Autodesk Inventor part; units mm, degrees
ref_plane "YZ Plane" through (0, 0, 0) normal (1, 0, 0) x (0, 1, 0)
ref_plane "XZ Plane" through (0, 0, 0) normal (0, 1, 0) x (-1, 0, 0)
ref_plane "XY Plane" through (0, 0, 0) normal (0, 0, 1) x (1, 0, 0)
sketch "Sketch4" plane through (0, 0, 0) normal (0, 0, 1) x (1, 0, 0)
  arc A0 (0.0635, 6.3497) -> (6.3497, 0.0635) centre (0, 0) ccw
  arc A1 (-1.1235, 7.5367) -> (7.5367, -1.1235) centre (0, 0) ccw
  line L0 (0, 0) -> (0, 7.9375) construction
  line L1 (0.0635, 6.3497) -> (6.3497, 0.0635) construction
  line L2 (0.0635, 6.3497) -> (-1.1235, 7.5367)
  line L3 (6.3497, 0.0635) -> (7.5367, -1.1235)
  circle A2 centre (0, 0) radius 6.35
  dimension "d10" = 12.7
  dimension "d11" = 1.27
  dimension "d12" = 45
  dimension "d13" = 8.89
extrude "Extrusion3" add sketch "Sketch4" along normal mid plane 35.56 contours A0 L3 A1 L2
sketch "Sketch5" plane through (0, 0, 0) normal (0, 0, 1) x (1, 0, 0)
  arc A0 (-1.1235, 7.5367) -> (7.5367, -1.1235) centre (0, 0) ccw
  line L0 (-7.62, 0) -> (-7.62, -29.21)
  line L1 (-7.62, -29.21) -> (0, -29.21)
  line L2 (0, -29.21) -> (0, -7.62)
  circle A1 centre (0, 0) radius 7.9375
  dimension "d16" = 21.59
extrude "Extrusion4" add sketch "Sketch5" along normal mid plane 35.56 contours A0 L2 A1 L0 | A1 L2 L1 L0 picked at (-7.3048, -2.4081)
sketch "Sketch6" plane through (0, -29.21, 17.78) normal (1, 0, 0) x (0, 0, -1)
  line L0 (0, 21.59) -> (35.56, 21.59)
  line L1 (35.56, 21.59) -> (35.56, 0)
  line L2 (0, 0) -> (35.56, 0)
  line L3 (0, 0) -> (0, 21.59)
  line L4 (17.78, 0) -> (17.78, 21.59) construction
  point P0 (17.78, 29.21)
  point P1 (17.78, 5.08)
  dimension "d30" = 5.08
  dimension "d31" = 0
hole "Hole1" at (0, -24.13, 0) direction (-1, 0, 0) diameter 3.5052 end through all countersink diameter 7.112 countersink angle 82
sketch "Sketch10" plane through (-7.62, -29.21, 17.78) normal (0, -1, 0) x (1, 0, 0)
  line L0 (0, -35.56) -> (0, 0)
  line L1 (7.62, -35.56) -> (0, -35.56)
  line L2 (7.62, 0) -> (7.62, -35.56)
  line L3 (0, 0) -> (7.62, 0)
  line L4 (3.81, -35.56) -> (3.81, 0) construction
  line L5 (6.35, -29.5599) -> (1.27, -29.5599)
  line L6 (1.27, -29.5599) -> (1.27, -26.3818)
  line L7 (1.27, -26.3818) -> (1.871, -26.3818)
  line L8 (1.871, -26.3818) -> (1.871, -28.8848)
  line L9 (1.871, -28.8848) -> (3.2625, -28.8848)
  line L10 (3.2625, -28.8848) -> (3.2625, -26.5506)
  line L11 (3.2625, -26.5506) -> (3.8635, -26.5506)
  line L12 (3.8635, -26.5506) -> (3.8635, -28.8848)
  line L13 (3.8635, -28.8848) -> (5.749, -28.8848)
  line L14 (5.749, -28.8848) -> (5.749, -26.3818)
  line L15 (5.749, -26.3818) -> (6.35, -26.3818)
  line L16 (6.35, -26.3818) -> (6.35, -29.5599)
  line L17 (1.27, -19.9474) -> (6.35, -21.2236)
  line L18 (6.35, -21.2236) -> (6.35, -21.9811)
  line L19 (6.35, -21.9811) -> (2.1345, -23.0144)
  line L20 (2.1345, -23.0144) -> (6.35, -24.0188)
  line L21 (6.35, -24.0188) -> (6.35, -24.7681)
  line L22 (6.35, -24.7681) -> (1.27, -26.0648)
  line L23 (1.27, -26.0648) -> (1.27, -25.3691)
  line L24 (1.27, -25.3691) -> (5.4814, -24.3482)
  line L25 (5.4814, -24.3482) -> (1.27, -23.3355)
  line L26 (1.27, -23.3355) -> (1.27, -22.648)
  line L27 (1.27, -22.648) -> (5.5308, -21.6271)
  line L28 (5.5308, -21.6271) -> (1.27, -20.6102)
  line L29 (1.27, -20.6102) -> (1.27, -19.9474)
  line L30 (4.4357, -17.6256) -> (4.4357, -19.5481)
  line L31 (4.4357, -19.5481) -> (3.8182, -19.5481)
  line L32 (3.8182, -19.5481) -> (3.8182, -17.6256)
  line L33 (3.8182, -17.6256) -> (4.4357, -17.6256)
  spline S0 degree 2 poles (2.8014, -13.5954) (3.1307, -13.5954) (3.7235, -13.83) (3.9294, -14.04) knots 0 0 0 1 2 2 2
  spline S1 degree 2 poles (3.9294, -14.04) (4.1887, -14.3035) (4.4563, -15.0156) (4.4563, -15.559) knots 0 0 0 1 2 2 2
  line L34 (4.4563, -15.559) -> (4.4563, -16.1313)
  line L35 (4.4563, -16.1313) -> (6.35, -16.1313)
  line L36 (6.35, -16.1313) -> (6.35, -16.8064)
  line L37 (6.35, -16.8064) -> (1.27, -16.8064)
  line L38 (1.27, -16.8064) -> (1.27, -15.5302)
  spline S2 degree 2 poles (1.27, -15.5302) (1.27, -15.0774) (1.4182, -14.4434) (1.587, -14.2005) knots 0 0 0 1 2 2 2
  spline S3 degree 2 poles (1.587, -14.2005) (1.7805, -13.9165) (2.3774, -13.5954) (2.8014, -13.5954) knots 0 0 0 1 2 2 2
  spline S4 degree 2 poles (2.822, -14.2993) (2.5585, -14.2993) (2.1716, -14.4805) (2.0481, -14.6657) knots 0 0 0 1 2 2 2
  spline S5 degree 2 poles (2.0481, -14.6657) (1.941, -14.8263) (1.8546, -15.2544) (1.8546, -15.5714) knots 0 0 0 1 2 2 2
  line L39 (1.8546, -15.5714) -> (1.8546, -16.1313)
  line L40 (1.8546, -16.1313) -> (3.88, -16.1313)
  line L41 (3.88, -16.1313) -> (3.88, -15.6702)
  spline S6 degree 2 poles (3.88, -15.6702) (3.88, -15.2585) (3.7482, -14.7522) (3.5753, -14.5875) knots 0 0 0 1 2 2 2
  spline S7 degree 2 poles (3.5753, -14.5875) (3.423, -14.4352) (3.0649, -14.2993) (2.822, -14.2993) knots 0 0 0 1 2 2 2
  line L42 (1.27, -9.2687) -> (6.35, -11.0183)
  line L43 (6.35, -11.0183) -> (6.35, -11.747)
  line L44 (6.35, -11.747) -> (1.27, -13.4966)
  line L45 (1.27, -13.4966) -> (1.27, -12.772)
  line L46 (1.27, -12.772) -> (5.4896, -11.3641)
  line L47 (5.4896, -11.3641) -> (1.27, -9.9562)
  line L48 (1.27, -9.9562) -> (1.27, -9.2687)
  line L49 (6.35, -5.9918) -> (6.35, -8.4701)
  line L50 (6.35, -8.4701) -> (5.8313, -8.4701)
  line L51 (5.8313, -8.4701) -> (5.8313, -7.548)
  line L52 (5.8313, -7.548) -> (2.4268, -7.548)
  line L53 (2.4268, -7.548) -> (2.4268, -8.4701)
  line L54 (2.4268, -8.4701) -> (1.9616, -8.4701)
  spline S8 degree 2 poles (1.9616, -8.4701) (1.9616, -7.9473) (1.6652, -7.4533) (1.2535, -7.4203) knots 0 0 0 1 2 2 2
  line L55 (1.2535, -7.4203) -> (1.2535, -6.8934)
  line L56 (1.2535, -6.8934) -> (5.8313, -6.8934)
  line L57 (5.8313, -6.8934) -> (5.8313, -5.9918)
  line L58 (5.8313, -5.9918) -> (6.35, -5.9918)
  point P0 (7.62, -17.78)
extrude "Text" cut sketch "Sketch10" against normal blind 1.143 contours L5 L6 L7 L8 L9 L10 L11 L12 L13 L14 L15 L16 | L17 L18 L19 L20 L21 L22 L23 L24 L25 L26 L27 L28 L29 | L30 L31 L32 L33 | S0 S1 L34 L35 L36 L37 L38 S2 S3 | L42 L43 L44 L45 L46 L47 L48 | L49 L50 L51 L52 L53 L54 S8 L55 L56 L57 L58
equation "\"d10\" = shadeDiameter"
equation "\"d11\" = shadeHolderWallThickness"
equation "\"d13\" = openingForShade"
equation "\"d14\" = partWidth"
equation "\"d16\" = flatBelowShade"
equation "\"d17\" = partWidth"
equation "\"d28\" = textDepth"
equation "\"shadeDiameter\" = 12.7"
equation "\"partWidth\" = 35.56"
equation "\"backThickness\" = 1.905"
equation "\"backHeight\" = 25.4"
equation "\"cutTiltAngle\" = 45deg"
equation "\"flatBelowShade\" = 21.59"
equation "\"shadeHolderWallThickness\" = 1.27"
equation "\"openingForShade\" = 8.89"
equation "\"textDepth\" = 1.143"
equation "\"holeHeightAboveBottom\" = 5.08"
properties part number "shadeHolderEmergencyExitWindow"
Verification items for the finished model (mm, model axes). A direction names the side the tool comes from. Give positions to 0.01 mm unless a question says otherwise; leave off trailing zeros. Write each loop counter-clockwise with the first axis right and the second up, starting at its lowest first coordinate (ties: lowest second). Pieces come first, ordered by that corner, then holes. Notation, with made-up numbers: (82.5, 65.5) - (128.5, 65.5) arc R10 cw to (128.5, 69.5) - close; hole circle Ø4 at (30.5, -26). An arc over 180 degrees is marked (long way). Answer as CSV lines item,"result". Start each with the question number.
1. Sectioned sample at A-A (y = -5.5). Record the boundary of the cut face in (x, z).
2. Depth check by flat-ended pin: pin 1 (0.6 mm diameter, centred on y = -28.5, z = 8, fed in from +X); pin 2 (2 mm diameter, centred on x = 0.5, z = -13, fed in from +Y); pin 3 (6 mm diameter, centred on x = -2, y = -2, fed in from -Z); pin 4 (2 mm diameter, centred on x = 4, z = -14, fed in from -Y). Enter the tip coordinate at first touch or a pass-through.
3. Set-up check for faces 1 (the face through (-4.19, -28.647, -3.346)), 2 (the face through (6.935, -0.522, -0.249)): record each of +Z, -Z, +X, -X, +Y, -Y from which the full face is reachable in a straight line by a thin tool's end or side.
4. Sectioned sample at B-B (z = -14). Record the boundary of the cut face in (x, y).
5. Sectioned sample at C-C (y = -11.5). Record the boundary of the cut face in (x, z), then the cut area to 3 significant figures.
6. Draft check along X on faces 3 (the face through (-1.945, -22.557, -1.003)), 4 (the face through (-3, -29, -11.105)), 5 (the face through (-4.21, -28.65, 7.11)). Enter one of: pulls with the +X half, pulls with the -X half, needs draft (parallel to the pull), parting line crosses it, or undercut.
7. Thickness scan on line 1 (Z direction, x = -4.55, y = -24.13); line 2 (Y direction, x = -3.5, z = -1); line 3 (Y direction, x = -3.25, z = 9). Record the ranges inside material, lowest first.
8. Sectioned sample at D-D (x = 4.75). Record the boundary of the cut face in (y, z).
Derived:
1,outline,"(-7.62, -17.78) - (-3.17, -17.78) - (-3.17, 17.78) - (-7.62, 17.78) - close; (3.17, -17.78) - (5.27, -17.78) - (5.27, 17.78) - (3.17, 17.78) - close"
2,pin 1,"x = 0"
2,pin 2,"y = 6.91"
2,pin 3,"through"
2,pin 4,"y = -7"
3,face 1,"-Y"
3,face 2,"+Z, -Z, +X, +Y"
4,outline,"(-7.62, -29.21) - (0, -29.21) - (0, -7.62) arc R7.62 ccw to (7.54, -1.12) - (6.35, 0.06) arc R6.35 cw (long way) to (0.06, 6.35) - (-1.12, 7.54) arc R7.62 ccw to (-7.62, 0) - close"
5,outline,"(-7.62, -17.78) - (0, -17.78) - (0, 17.78) - (-7.62, 17.78) - close"
5,area,"271 mm²"
6,face 3,"pulls with the +X half"
6,face 4,"undercut"
6,face 5,"undercut"
7,line 1,"-17.78 to -1.75, 1.75 to 17.78"
7,line 2,"-28.07 to -25.57, -22.69 to -5.3, 5.3 to 6.77"
7,line 3,"-29.21 to -5.46, 5.46 to 6.89"
8,outline,"(-5.96, -17.78) - (-4.21, -17.78) - (-4.21, 17.78) - (-5.96, 17.78) - close"
